```python
from build123d import *

# Parameters (mm, degrees)
SKETCH1_R               = 25.4
BOSS_EXTRUDE1_DEPTH     = 9.525
SKETCH2_W               = 19.05
SKETCH2_H               = 19.05
BOSS_EXTRUDE2_DEPTH     = 28.575
SKETCH3_R               = 19.05
CUT_EXTRUDE1_DEPTH      = 43.715256349
CUT_EXTRUDE2_REACH      = 62.408
CUT_EXTRUDE2_END_RADIUS = 19.05
SKETCH4_R               = 4.826


with BuildPart() as part:
    # Sketch1 → Boss-Extrude1 (new, symmetric)
    with BuildSketch(Plane.XY):
        with Locations(Location((0, 0, 0), (0, 0, 180))):
            Circle(SKETCH1_R)
    extrude(amount=BOSS_EXTRUDE1_DEPTH, both=True)

    # Sketch2 → Boss-Extrude2 (add)
    with BuildSketch(Plane(origin=(0, 0, 0), x_dir=(1, 0, 0), z_dir=(0, 1, 0))):
        Rectangle(SKETCH2_W, SKETCH2_H)
    extrude(amount=BOSS_EXTRUDE2_DEPTH)

    # Sketch3 → Cut-Extrude1 (cut, through all)
    with BuildSketch(Plane.XY.offset(9.525)):
        Circle(SKETCH3_R)
    extrude(amount=-CUT_EXTRUDE1_DEPTH, mode=Mode.SUBTRACT)

    # Cut-Extrude2: up to this cylinder (the profile starts outside it)
    cut_extrude2_end = Plane(origin=(0, 0, 0), z_dir=(0, 0, 1)) * Cylinder(CUT_EXTRUDE2_END_RADIUS, 163.916, mode=Mode.PRIVATE)
    # Sketch4 → Cut-Extrude2 (cut, up to the surface)
    with BuildSketch(Plane(origin=(0, 28.575, 0), x_dir=(1, 0, 0), z_dir=(0, 1, 0)), mode=Mode.PRIVATE) as cut_extrude2_sk1:
        with Locations(Location((0, 0, 0), (0, 0, 270))):
            Circle(SKETCH4_R)
    cut_extrude2_tool1 = extrude(cut_extrude2_sk1.sketch, amount=-CUT_EXTRUDE2_REACH, mode=Mode.PRIVATE) - cut_extrude2_end
    add(cut_extrude2_tool1.solids().sort_by_distance((0, 28.575, 0))[0], mode=Mode.SUBTRACT)


solid = part.part
```
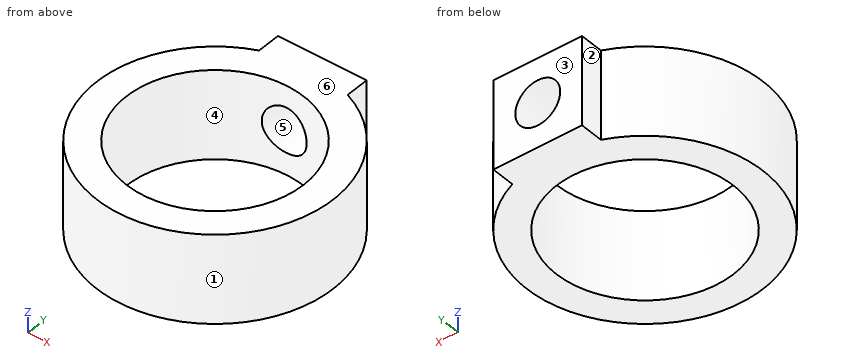
Source: CAD feature listing. Evaluate the final solid. Frame: model axes, mm. Face numbers are marked on the shaded views. A direction names the side the tool comes from. Coordinates: 2 decimals unless noted, no trailing zeros. Write each loop counter-clockwise with the first axis right and the second up, starting at its lowest first coordinate (ties: lowest second). Pieces come first, ordered by that corner, then holes. Notation, with made-up numbers: (-35.5, -40) -> (18.5, -40) arc R36 ccw to (18.5, -3) -> close; hole circle Ø2 at (-22, -12.75). An arc over 180 degrees is marked (long way). Return JSON: item names as keys, results as strings. Group by question number.
1) Ray query, line 1 along Y through (x, z) = (-3, 5.5) (3 decimals); line 2 along Z through (x, y) = (0, 26.5) (3 decimals); line 3 along X through (y, z) = (-14, 3.5). Return the intervals inside material, ascending.
2) Mould query, pull axis Y, two halves, no side actions, for the marked faces 1, 2, 3 and 4. Classes: +Y half, -Y half, draft (parallel to the pull), parting line (faces both ways), or undercut.
3) Section query B-B, the plane x = 0. Return loops of the section in (y, z) (3 decimals).
4) Section query A-A, the plane y = 0. Return loops of the section in (x, z) (3 decimals).
5) Section query C-C, the plane z = 0. Return loops of the section in (x, y) (3 decimals), plus the area to 3 significant figures.
6) Contact query for flat-ended pins moving along their axis: P1, Ø5, axis at x = 12, z = -4.5, coming from the -Y side; P2, Ø2, axis at x = 7, z = -6, coming from the -Y side; P3, Ø2.5, axis at y = 27, z = -3.5, coming from the +X side (3 decimals); P4, Ø23, axis at x = 0, y = 0, coming from the +Z side. Output: stop coordinate, or through.
7) Section query D-D, the plane x = -5.5. Return loops of the section in (y, z) (3 decimals), plus the area to 3 significant figures.
8) Set-up query: the marked faces 5 and 6. Return all of +Z, -Z, +X, -X, +Y, -Y with unobstructed straight access to the full face (end or side cutting, diameter ignored); none if empty.
From the geometry:
{
 "1": {"line 1": "-25.222 to -18.812, 18.812 to 28.575", "line 2": "-9.525 to -4.826, 4.826 to 9.525", "line 3": "-21.19 to -12.92, 12.92 to 21.19"},
 "2": {"face 1": "parting line", "face 2": "draft", "face 3": "+Y half", "face 4": "undercut"},
 "3": {"outline": "(-25.4, -9.525) -> (-19.05, -9.525) -> (-19.05, 9.525) -> (-25.4, 9.525) -> close; (19.05, -9.525) -> (28.575, -9.525) -> (28.575, -4.826) -> (19.05, -4.826) -> close; (19.05, 4.826) -> (28.575, 4.826) -> (28.575, 9.525) -> (19.05, 9.525) -> close"},
 "4": {"outline": "(-25.4, -9.525) -> (-19.05, -9.525) -> (-19.05, 9.525) -> (-25.4, 9.525) -> close; (19.05, -9.525) -> (25.4, -9.525) -> (25.4, 9.525) -> (19.05, 9.525) -> close"},
 "5": {"outline": "(-9.525, 23.546) arc R25.4 ccw (long way) to (9.525, 23.546) -> (9.525, 28.575) -> (4.826, 28.575) -> (4.826, 18.429) arc R19.05 cw (long way) to (-4.826, 18.429) -> (-4.826, 28.575) -> (-9.525, 28.575) -> close", "area": "865 mm²"},
 "6": {"P1": "y = -23.56", "P2": "y = -24.68", "P3": "x = 9.525", "P4": "through"},
 "7": {"outline": "(-24.797, -9.525) -> (-18.239, -9.525) -> (-18.239, 9.525) -> (-24.797, 9.525) -> close; (18.239, -9.525) -> (28.575, -9.525) -> (28.575, 9.525) -> (18.239, 9.525) -> close", "area": "322 mm²"},
 "8": {"face 5": "+Y", "face 6": "+Z, +X, -X, +Y, -Y"}
}
